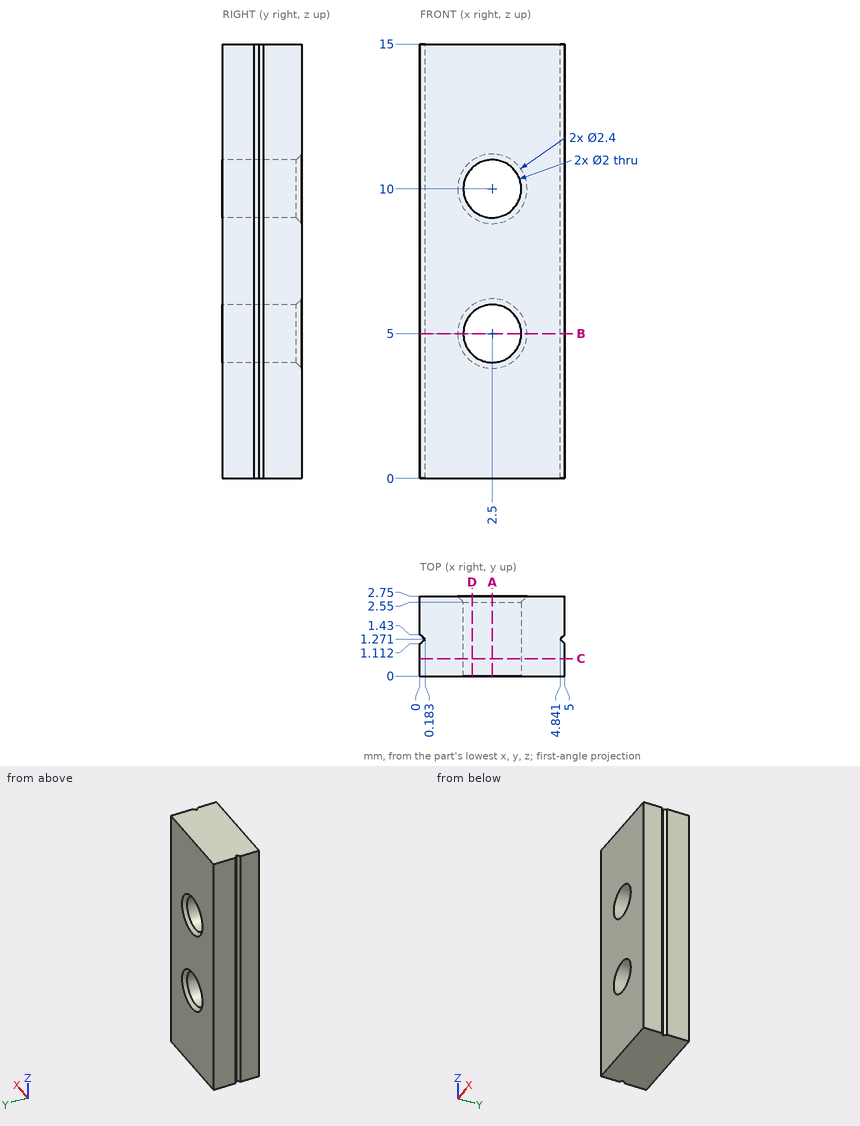
Geometry check sheet. Reference: drawing and pictorial views, mm from the part's lowest x, y, z. Round coordinates to 2 decimals unless told otherwise and drop trailing zeros. Order: outer loops, then holes, each group sorted by start corner. A loop starts at its lowest first (then second) coordinate and runs counter-clockwise, first axis right, second up. Notation, with made-up numbers: M 16,5.5 L 42,5.5 A15 ccw 42,31.5 Z; hole C 83,40 d3. An arc over 180 degrees is marked long. One line per item, written item: value. Start each with the question number.
1. Section check A-A on x = 2.5. Enter the section's corners in (y, z).
2. Section check B-B on z = 5. Enter the section's corners in (x, y).
3. Section check D-D on x = 1.8. Give the number of separate pieces and of enclosed holes in the cut face, and give its area (3 significant figures).
4. Scan lines: line 1 along Z through (x, y) = (2.5, 1); line 2 along X through (y, z) = (1.85, 5); line 3 along X through (y, z) = (1.2, 5). Record each from-to range of solid material in increasing order.
5. Section check C-C on y = 0.6. Enter the section's corners in (x, z).
Results found:
1. outline: M 0,0 L 2.75,0 L 2.75,3.8 L 2.55,4 L 0,4 Z; M 0,6 L 2.55,6 L 2.75,6.2 L 2.75,8.8 L 2.55,9 L 0,9 Z; M 0,11 L 2.55,11 L 2.75,11.2 L 2.75,15 L 0,15 Z
2. outline: M 0,0 L 1.5,0 L 1.5,2.55 L 1.3,2.75 L 0,2.75 L 0,1.43 L 0.18,1.27 L 0,1.11 Z; M 3.5,0 L 5,0 L 5,1.11 L 4.84,1.27 L 5,1.43 L 5,2.75 L 3.7,2.75 L 3.5,2.55 Z
3. separate pieces: 3
3. enclosed holes: 0
3. area: 33.3 mm^2
4. line 1: 0 to 4, 6 to 9, 11 to 15
4. line 2: 0 to 1.5, 3.5 to 5
4. line 3: 0.1 to 1.5, 3.5 to 4.91
5. outline: M 0,0 L 5,0 L 5,15 L 0,15 Z; hole C 2.5,5 d2; hole C 2.5,10 d2
